```python
from build123d import *

# Parameters (mm, degrees)
F0_R     = 46
F1_DEPTH = 25
F3_DEPTH = 10
F4_W     = 77
F4_H     = 13
F5_DEPTH = 15


with BuildPart() as f1:
    # F0 (on Top) → F1 (new body)
    with BuildSketch(Plane.XY):
        Circle(F0_R)
    extrude(amount=F1_DEPTH)

    # F2 (on face) → F3 (cut)
    with BuildSketch(Plane(origin=(0, 0, 0), x_dir=(1, 0, 0), z_dir=(0, 0, -1))):
        with BuildLine():
            Line((29.344931, -29.344931), (26.516504, -26.516504))
            ThreePointArc((26.516504, -26.516504), (0, 37.5), (-26.516504, -26.516504))
            Line((-26.516504, -26.516504), (-29.344931, -29.344931))
            ThreePointArc((-29.344931, -29.344931), (0, -41.5), (29.344931, -29.344931))
        make_face()
    extrude(amount=-F3_DEPTH, mode=Mode.SUBTRACT)

    # F4 (on face) → F5 (cut)
    with BuildSketch(Plane.XY.offset(25)):
        Rectangle(F4_W, F4_H)
    extrude(amount=-F5_DEPTH, mode=Mode.SUBTRACT)


solid = f1.part
```
Here's how the part is built. I have some questions about the finished solid (model axes, mm). A direction names the side the tool comes from. Give positions to 0.01 mm unless a question says otherwise; leave off trailing zeros. Write each loop counter-clockwise with the first axis right and the second up, starting at its lowest first coordinate (ties: lowest second). Pieces come first, ordered by that corner, then holes. Notation, with made-up numbers: M -23,30.5 L 20,30.5 A34 cw 20,69.5 Z; hole C -23,84.5 d5. An arc over 180 degrees is marked long. Put each result on its own line as item: value. Start each with the question number.
Item 1: I need wall thicknesses on L1, parallel to Y at x = -1, z = 14; L2, parallel to Y at x = 0, z = 5; L3, parallel to Z at x = 8, y = 30. Which ranges of each line are inside material? Lowest first, please. Write a range as from..to.
Item 2: If we section it at B-B, the plane z = 8.5: Write out the boundary of the cut face in (x, y), then the cut area to 3 significant figures.
Item 3: If we section it at D-D, the plane y = 24: Write out the boundary of the cut face in (x, z).
Item 4: Will these pins go through, and if not, where does the flat tip stop? pin 1 (1 mm diameter, centred on y = 19.5, z = 4.5, fed in from -X); pin 2 (10 mm diameter, centred on x = 31, z = 14, fed in from -Y); pin 3 (12 mm diameter, centred on x = -3.5, z = 17, fed in from -Y).
Item 5: Thinking about a two-plate mould opening in Y: for faces 3 (the flat face through (-38.5, 0, 18)), 4 (the flat face through (-1, -10, 25)), 5 (the flat face through (38.5, 0, 18)), 6 (the cylindrical face through (-5.99, 45.61, 12.32)), which applies, +Y half, -Y half, draft (parallel to the pull), parting line (faces both ways), or undercut?
Item 6: On a 3-axis mill with a long thin cutter (end or side, diameter ignored), from which of +Z, -Z, +X, -X, +Y, -Y can I reach the whole of each face in a straight line? I mean faces 1 (the flat face through (-7, -37, 0)), 2 (the flat face through (-28, 28, 5)). Say none if no direction works.
Item 7: If we section it at C-C, the plane x = 0: Write out the boundary of the cut face in (y, z), then the cut area to 4 significant figures.
Item 8: If we section it at A-A, the plane y = 0: Write out the boundary of the cut face in (x, z), then the cut area to 3 significant figures.
Values:
1. L1: -45.99..-6.5, 6.5..45.99
1. L2: -46..-37.5, 41.5..46
1. L3: 10..25
2. outline: C 0,0 d92; hole M -29.34,29.34 L -26.52,26.52 A37.5 ccw long 26.52,26.52 L 29.34,29.34 A41.5 ccw Z
2. area: 1,980 mm²
3. outline: M -39.24,0 L -28.81,0 L -28.81,10 L 28.81,10 L 28.81,0 L 39.24,0 L 39.24,25 L -39.24,25 Z
4. pin 1: x = -41.89
4. pin 2: y = -37.95
4. pin 3: y = -46
5. face 3: undercut
5. face 4: draft
5. face 5: undercut
5. face 6: parting line
6. face 1: -Z, +X, -X, +Y, -Y
6. face 2: -Z
7. outline: M -46,0 L -37.5,0 L -37.5,10 L -6.5,10 L -6.5,25 L -46,25 Z; M 6.5,10 L 41.5,10 L 41.5,0 L 46,0 L 46,25 L 6.5,25 Z
7. area: 1,315 mm²
8. outline: M -46,0 L -37.5,0 L -37.5,10 L -38.5,10 L -38.5,25 L -46,25 Z; M 37.5,0 L 46,0 L 46,25 L 38.5,25 L 38.5,10 L 37.5,10 Z
8. area: 395 mm²
